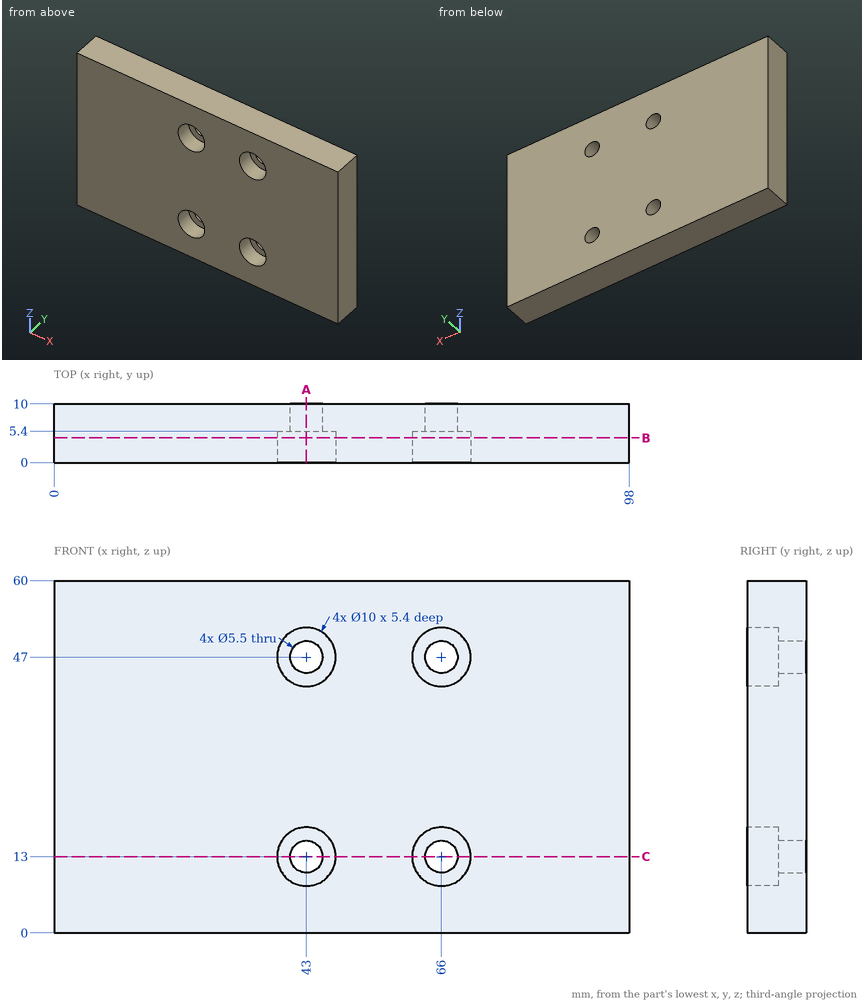
Job drawing, mm, ordinate dimensions from the low corner. One solid piece. Give positions to 0.01 mm unless a question says otherwise; leave off trailing zeros. Order: outer loops, then holes, each group sorted by start corner. A loop starts at its lowest first (then second) coordinate and runs counter-clockwise, first axis right, second up. Notation, with made-up numbers: M 58,50 L 74,50 A14 ccw 74,57 Z; hole C -30,58.25 d4. An arc over 180 degrees is marked long. Return JSON: item names as keys, results as strings.
Q1. Wall check: probe 1 along Z at (x, y) = (66, 6.8); probe 2 along X at (y, z) = (2.75, 13); probe 3 along X at (y, z) = (8.6, 13). Give the ranges that are in metal, low to high. Write a range as from..to.
Answer list:
{"probe 1": "z = 0..10.25, 15.75..44.25, 49.75..60", "probe 2": "x = 0..38, 48..61, 71..98", "probe 3": "x = 0..40.25, 45.75..63.25, 68.75..98"}
Q2. Band-saw the part on C-C (z = 13). Give the cut face in (x, y).
Answer list:
{"outline": "M 0,0 L 38,0 L 38,5.4 L 40.25,5.4 L 40.25,10 L 0,10 Z; M 45.75,5.4 L 48,5.4 L 48,0 L 61,0 L 61,5.4 L 63.25,5.4 L 63.25,10 L 45.75,10 Z; M 68.75,5.4 L 71,5.4 L 71,0 L 98,0 L 98,10 L 68.75,10 Z"}
Q3. Band-saw the part on B-B (y = 4.25). Give the cut face in (x, z), then the cut area to 3 significant figures.
Answer list:
{"outline": "M 0,0 L 98,0 L 98,60 L 0,60 Z; hole C 43,13 d10; hole C 43,47 d10; hole C 66,13 d10; hole C 66,47 d10", "area": "5,570 mm^2"}
Q4. Flat gauge pins, fed straight in: pin 1 (3.5 mm diameter, centred on x = 43, z = 13, fed in from -Y); pin 2 (6 mm diameter, centred on x = 43, z = 47, fed in from -Y). Where does each tip first touch, or does it go through?
Answer list:
{"pin 1": "passes through", "pin 2": "stops at y = 5.4"}
Q5. Band-saw the part on A-A (x = 43). Give the cut face in (y, z).
Answer list:
{"outline": "M 0,0 L 10,0 L 10,10.25 L 5.4,10.25 L 5.4,8 L 0,8 Z; M 0,18 L 5.4,18 L 5.4,15.75 L 10,15.75 L 10,44.25 L 5.4,44.25 L 5.4,42 L 0,42 Z; M 0,52 L 5.4,52 L 5.4,49.75 L 10,49.75 L 10,60 L 0,60 Z"}
